from build123d import *

# Parameters (mm, degrees)
BOSS_EXTRUDE1_DEPTH = 20
SKETCH2_R           = 5
CUT_EXTRUDE1_DEPTH  = 41


with BuildPart() as part:
    # Sketch1 → Boss-Extrude1 (new body)
    with BuildSketch(Plane(origin=(0, 0, 0), x_dir=(1, 0, 0), z_dir=(0, 1, 0))):
        with BuildLine():
            ThreePointArc((-34.641016151, -20), (-38.637033052, -10.352761804), (-40, 0))
            Line((-40, 0), (-45, 0))
            Line((-45, 0), (-45, -20))
            Line((-45, -20), (-34.641016151, -20))
        make_face()
        with BuildLine():
            Line((40, 0), (15, 0))
            ThreePointArc((15, 0), (0, -15), (-15, 0))
            Line((-15, 0), (-40, 0))
            ThreePointArc((-40, 0), (-38.637033052, -10.352761804), (-34.641016151, -20))
            Line((-34.641016151, -20), (34.641016151, -20))
            ThreePointArc((34.641016151, -20), (38.637033052, -10.352761804), (40, 0))
        make_face()
        with BuildLine():
            ThreePointArc((-34.641016151, -20), (0, -40), (34.641016151, -20))
            Line((34.641016151, -20), (-34.641016151, -20))
        make_face()
        with BuildLine():
            Line((45, 0), (40, 0))
            ThreePointArc((40, 0), (38.637033052, -10.352761804), (34.641016151, -20))
            Line((34.641016151, -20), (45, -20))
            Line((45, -20), (45, 0))
        make_face()
    extrude(amount=BOSS_EXTRUDE1_DEPTH)

    # Sketch2 → Cut-Extrude1 (cut, through all)
    with BuildSketch(Plane(origin=(0, 0, 0), x_dir=(-1, 0, 0), z_dir=(0, 0, -1))):
        with Locations((-35, 10)):
            Circle(SKETCH2_R)
        with Locations((35, 10)):
            Circle(SKETCH2_R)
    extrude(amount=-CUT_EXTRUDE1_DEPTH, mode=Mode.SUBTRACT)


solid = part.part
Geometry check sheet. Reference: the model listing, model coordinates, mm. A direction names the side the tool comes from. Give positions to 0.01 mm unless a question says otherwise; leave off trailing zeros. Order: outer loops, then holes, each group sorted by start corner. A loop starts at its lowest first (then second) coordinate and runs counter-clockwise, first axis right, second up.
1. Depth check by flat-ended pin: pin 1 (11.5 mm diameter, centred on x = -35, y = 10, fed in from +Z); pin 2 (4 mm diameter, centred on x = -27.5, y = 7, fed in from +Z); pin 3 (2 mm diameter, centred on y = 13.5, z = 30.5, fed in from -X). Enter the tip coordinate at first touch or a pass-through.
Completed:
pin 1: stops at z = 27.28
pin 2: stops at z = 30.82
pin 3: stops at x = -27.01
2. Sectioned sample at C-C (y = 2). Record the boundary of the cut face in (x, z).
Completed:
outline: (-45, 0) - (-15, 0) arc R15 cw to (15, 0) - (45, 0) - (45, 20) - (34.64, 20) arc R40 ccw to (-34.64, 20) - (-45, 20) - close
3. Scan lines: line 1 (Y direction, x = 35, z = 16); line 2 (X direction, y = 10, z = 5.75); line 3 (X direction, y = 10, z = 11.25). Record each from-to range of solid material in increasing order.
Completed:
line 1: y = 0 to 5, 15 to 20
line 2: x = -45 to -40, -30 to -13.85, 13.85 to 30, 40 to 45
line 3: x = -45 to -40, -30 to -9.92, 9.92 to 30, 40 to 45
4. Sectioned sample at A-A (z = 13). Record the boundary of the cut face in (x, y).
Completed:
outline: (-45, 0) - (-7.48, 0) - (-7.48, 20) - (-45, 20) - close; (7.48, 0) - (45, 0) - (45, 20) - (7.48, 20) - close; hole circle Ø10 at (-35, 10); hole circle Ø10 at (35, 10)
5. Sectioned sample at B-B (y = 10). Record the boundary of the cut face in (x, z), then the cut area to 3 significant figures.
Completed:
outline: (-45, 0) - (-40, 0) - (-40, 20) - (-45, 20) - close; (-30, 0) - (-15, 0) arc R15 cw to (15, 0) - (30, 0) - (30, 26.46) arc R40 ccw to (-30, 26.46) - close; (40, 0) - (45, 0) - (45, 20) - (40, 20) - close
area: 2,000 mm2
6. Access from +Z, -Z, +X, -X, +Y, -Y to the whole of each face (thin tool, end or side, straight path). Record for faces 1 (the face through (41, 10, 20)), 2 (the face through (-41, 10, 20)), 3 (the face through (-30, 10, 10)).
Completed:
face 1: +Z, +X, +Y, -Y
face 2: +Z, -X, +Y, -Y
face 3: +Z, -Z
7. Draft check along X on faces 4 (the face through (-45, 10, 10)), 5 (the face through (-0.586, 9.86, 39.996)), 6 (the face through (30.23, 11.5, 10.1)). Enter one of: pulls with the +X half, pulls with the -X half, needs draft (parallel to the pull), parting line crosses it, or undercut.
Completed:
face 4: pulls with the -X half
face 5: parting line crosses it
face 6: undercut
8. Sectioned sample at D-D (z = 5). Record the boundary of the cut face in (x, y), then the cut area to 3 significant figures.
Completed:
outline: (-45, 0) - (-14.14, 0) - (-14.14, 20) - (-45, 20) - close; (14.14, 0) - (45, 0) - (45, 20) - (14.14, 20) - close; hole circle Ø10 at (-35, 10); hole circle Ø10 at (35, 10)
area: 1,080 mm2
